from build123d import *

# Parameters (mm, degrees)
F0_W     = 300.2
F0_H     = 110.2
F1_DEPTH = 5
F2_W     = 300.2
F2_H     = 9.9
F3_DEPTH = 0.8
F4_W     = 4.9
F4_H     = 9.8
F4_W_2   = 9.8
F4_H_2   = 4.9
F5_DEPTH = 5


with BuildPart() as f1:
    # F0 (on Front) → F1 (new body)
    with BuildSketch(Plane.XZ):
        Rectangle(F0_W, F0_H)
    extrude(amount=F1_DEPTH)

    # F2 (on face) → F3 (cut)
    with BuildSketch(Plane.XZ.offset(5)):
        with Locations((0, 50.15)):
            Rectangle(F2_W, F2_H)
    extrude(amount=-F3_DEPTH, mode=Mode.SUBTRACT)

    # F4 (on face) → F5 (cut, through all)
    with BuildSketch(Plane.XZ.offset(5)):
        with Locations((-147.65, 22.5)):
            Rectangle(F4_W, F4_H)
        with Locations((-147.65, -27.5)):
            Rectangle(F4_W, F4_H)
        with Locations((-100, -52.65)):
            Rectangle(F4_W_2, F4_H_2)
        with Locations((-50, -52.65)):
            Rectangle(F4_W_2, F4_H_2)
        with Locations((0, -52.65)):
            Rectangle(F4_W_2, F4_H_2)
        with Locations((50, -52.65)):
            Rectangle(F4_W_2, F4_H_2)
        with Locations((147.65, 22.5)):
            Rectangle(F4_W, F4_H)
        with Locations((147.65, -27.5)):
            Rectangle(F4_W, F4_H)
        with Locations((100, -52.65)):
            Rectangle(F4_W_2, F4_H_2)
    extrude(amount=-F5_DEPTH, mode=Mode.SUBTRACT)


solid = f1.part
Design review of the part built by this model. Coordinates are the model's own, in mm. A direction names the side the tool comes from. Round coordinates to 2 decimals unless told otherwise and drop trailing zeros. One line per item, written item: value. Start each with the question number.
Q1. The part is to be moulded in two halves that separate along Z. For faces 1 (the face through (148, -3, 27.4)), 2 (the face through (-104.9, -3, -53)), 3 (the face through (25, -2, -55.1)), say which applies: pulls with the +Z half, pulls with the -Z half, needs draft (parallel to the pull), parting line crosses it, or undercut.
Q2. Tool access review of faces 4 (the face through (100, -3, -50.2)), 5 (the face through (-148, -3, 27.4)), 6 (the face through (-2, -4.2, 50)), 7 (the face through (148, -3, 17.6)): name each direction out of +Z, -Z, +X, -X, +Y, -Y from which nothing blocks a thin tool from reaching the whole face with its end or side.
Q3. To check wall thickness, follow probe 1 along X at (y, z) = (-4.8, 24); probe 2 along Z at (x, y) = (4, -0.45); probe 3 along Y at (x, z) = (124, 49). State the ranges of each line that lie inside material, in increasing order.
Q4. Insertion check: P1, Ø2, axis at x = -52, y = -4, coming from the -Z side; P2, Ø6, axis at x = -44, z = -7, coming from the +Y side; P3, Ø1.5, axis at y = -3, z = 23.5, coming from the +X side. Each pin has a flat end and moves straight along its axis. Give the tip position at first contact, or say it passes through.
Response:
1. face 1: undercut
1. face 2: needs draft
1. face 3: pulls with the -Z half
2. face 4: -Z, +Y, -Y
2. face 5: -X, +Y, -Y
2. face 6: +Z, +X, -X, -Y
2. face 7: +X, +Y, -Y
3. probe 1: x = -145.2 to 145.2
3. probe 2: z = -50.2 to 55.1
3. probe 3: y = -4.2 to 0
4. P1: stops at z = -50.2
4. P2: stops at y = 0
4. P3: stops at x = 145.2
